Work out the finished part from the listing and answer in its coordinate system (mm). Face numbers are marked on the shaded views. A direction names the side the tool comes from. Give positions to 0.01 mm unless a question says otherwise; leave off trailing zeros. Loops run counter-clockwise (first coordinate to the right, second up) from the corner with the lowest first, then second, coordinate; pieces in that order, holes last. Notation, with made-up numbers: M -6.75,58.25 L 40.25,58.25 A24 cw 40.25,82.25 Z; hole C 5.5,-21 d5. An arc over 180 degrees is marked long. Use a Markdown table: item, result.
```python
from build123d import *

# Parameters (mm, degrees)
F2_DEPTH = 4
F4_DEPTH = 4
F5_W     = 129.927155
F5_H     = 119.906087
F5_W_2   = 40
F5_H_2   = 40
F6_DEPTH = 8.001


with BuildPart() as f2:
    # F1 (on Top) → F2 (new body)
    with BuildSketch(Plane.XY):
        Polygon((40.684865, -47.513555), (-21.115135, -47.513555), (-21.115135, 14.286445), (-40.215135, 33.386445), (-40.215135, -66.613555), (59.784865, -66.613555), align=None)
    extrude(amount=F2_DEPTH)

    # F3 (on face) → F4 (join)
    with BuildSketch(Plane.XY.offset(4)):
        Polygon((-24.115135, -3.086945), (-40.215135, -3.086945), (-40.215135, -66.613555), (15.733283, -66.613555), (15.733283, -50.513555), (-24.115135, -50.513555), align=None)
    extrude(amount=F4_DEPTH)

    # F5 (on Top) → F6 (cut, through all)
    with BuildSketch(Plane.XY):
        with Locations((8.65676, -20.336797)):
            Rectangle(F5_W, F5_H)
        with Locations((-7.115135, -33.513555)):
            Rectangle(F5_W_2, F5_H_2, mode=Mode.SUBTRACT)
    extrude(amount=F6_DEPTH, mode=Mode.SUBTRACT)


solid = f2.part
```
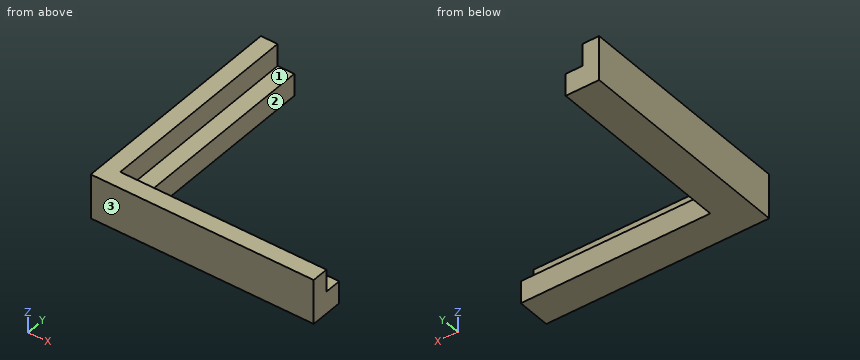
(1) A cutting plane is placed at A-A (z = 3). Write down the section's boundary in (x, y), and give its area (3 significant figures).
Entries:
| item | result |
|---|---|
| outline | M -27.12,-53.51 L 12.88,-53.51 L 12.88,-47.51 L -21.12,-47.51 L -21.12,-13.51 L -27.12,-13.51 Z |
| area | 444 mm² |
(2) Which of the six approach directions +Z, -Z, +X, -X, +Y, -Y give full straight-line access (tool end or side, diameter ignored) to the marked faces 1, 2 and 3?
Entries:
| item | result |
|---|---|
| face 1 | +Z, +X, +Y |
| face 2 | +Z, -Z, +X, +Y |
| face 3 | +Z, -Z, +X, -X, -Y |
(3) Consider probe 1 along Y at (x, z) = (0.5, 3.25); probe 2 along Z at (x, y) = (-23, -40); probe 3 along X at (y, z) = (-34, 5.75). Determine where each line is inside the solid, lowest interval first. Write a range as [from, to].
Entries:
| item | result |
|---|---|
| probe 1 | y = [-53.51, -47.51] |
| probe 2 | z = [0, 4] |
| probe 3 | x = [-27.12, -24.12] |
(4) Given P1, Ø3, axis at x = -20.5, z = 1, coming from the +Y side; P2, Ø4, axis at x = 1.5, z = 1.5, coming from the +Y side; P3, Ø4, axis at y = -45, z = 2.5, coming from the +X side; P4, Ø1.2, axis at x = -5.5, z = 6, coming from the +Y side, each flat-ended and moving along its own axis, determine where each tip first touches the part or whether it passes through.
Entries:
| item | result |
|---|---|
| P1 | stops at y = -13.51 |
| P2 | stops at y = -47.51 |
| P3 | stops at x = -21.12 |
| P4 | stops at y = -50.51 |
(5) A cutting plane is placed at B-B (y = -30.5). Write down the section's boundary in (x, z), and give its area (3 significant figures).
Entries:
| item | result |
|---|---|
| outline | M -27.12,0 L -21.12,0 L -21.12,4 L -24.12,4 L -24.12,8 L -27.12,8 Z |
| area | 36.0 mm² |
